Work out the finished part from the listing and answer in its coordinate system (mm). A direction names the side the tool comes from. Coordinates: 2 decimals unless noted, no trailing zeros. Order: outer loops, then holes, each group sorted by start corner. A loop starts at its lowest first (then second) coordinate and runs counter-clockwise, first axis right, second up. Notation, with made-up numbers: M 59.5,-24 L 108.5,-24 A21 cw 108.5,-18 Z; hole C -0.5,-25 d11. An arc over 180 degrees is marked long. Use a Markdown table: item, result. Add a question column.
from build123d import *

# Parameters (mm, degrees)
ESQUISSE1_W              = 86
ESQUISSE1_H              = 40
BOSS_EXTRU_1_DEPTH       = 4
ESQUISSE2_R              = 10.5
ENL_V_MAT_EXTRU_1_DEPTH  = 95.93155429
ESQUISSE3_W              = 6
ESQUISSE3_H              = 40
BOSS_EXTRU_2_DEPTH       = 120
ESQUISSE4_W              = 40
ESQUISSE4_H              = 5
BOSS_EXTRU_3_DEPTH       = 20
ESQUISSE5_W              = 40
ESQUISSE5_H              = 5
BOSS_EXTRU_4_DEPTH       = 20
D_GAGEMENT_M51_D         = 5.5
ESQUISSE32_W             = 40
ESQUISSE32_H             = 31
BOSS_EXTRU_5_DEPTH       = 29.5
ESQUISSE33_W             = 40
ESQUISSE33_H             = 31
BOSS_EXTRU_6_DEPTH       = 29.5
ESQUISSE39_R             = 1.5
ENL_V_MAT_EXTRU_4_DEPTH  = 168.964281917
ESQUISSE43_W             = 30
ESQUISSE43_H             = 31
ENL_V_MAT_EXTRU_12_DEPTH = 29.5
ESQUISSE44_W             = 30
ESQUISSE44_H             = 31
ENL_V_MAT_EXTRU_13_DEPTH = 29.5
ENL_V_MAT_EXTRU_14_DEPTH = 166.033329967
ESQUISSE47_R             = 1.75
ESQUISSE47_R_2           = 1.7
ENL_V_MAT_EXTRU_15_DEPTH = 168.964281917


with BuildPart() as part:
    # Esquisse1 → Boss.-Extru.1 (new body)
    with BuildSketch(Plane(origin=(0, 0, 0), x_dir=(1, 0, 0), z_dir=(0, 1, 0))):
        with Locations((43, 20)):
            Rectangle(ESQUISSE1_W, ESQUISSE1_H)
    extrude(amount=BOSS_EXTRU_1_DEPTH)

    # Esquisse2 → Enlèv. mat.-Extru.1 (cut, through all)
    with BuildSketch(Plane(origin=(0, 4, 0), x_dir=(1, 0, 0), z_dir=(0, 1, 0))):
        with Locations(Location((43, 20, 0), (0, 0, 270))):
            Circle(ESQUISSE2_R)
    extrude(amount=-ENL_V_MAT_EXTRU_1_DEPTH, mode=Mode.SUBTRACT)

    # Esquisse3 → Boss.-Extru.2 (add)
    with BuildSketch(Plane(origin=(0, 0, 0), x_dir=(-1, 0, 0), z_dir=(0, -1, 0))):
        with Locations((-3, 20)):
            Rectangle(ESQUISSE3_W, ESQUISSE3_H)
        with Locations((-83, 20)):
            Rectangle(ESQUISSE3_W, ESQUISSE3_H)
    extrude(amount=BOSS_EXTRU_2_DEPTH)

    # Esquisse4 → Boss.-Extru.3 (add)
    with BuildSketch(Plane.ZY):
        with Locations((-20, -117.5)):
            Rectangle(ESQUISSE4_W, ESQUISSE4_H)
    extrude(amount=BOSS_EXTRU_3_DEPTH)

    # Esquisse5 → Boss.-Extru.4 (add)
    with BuildSketch(Plane(origin=(86, 0, 0), x_dir=(0, 0, -1), z_dir=(1, 0, 0))):
        with Locations((20, -117.5)):
            Rectangle(ESQUISSE5_W, ESQUISSE5_H)
    extrude(amount=BOSS_EXTRU_4_DEPTH)

    # Dégagement M51 (through all)
    with Locations(Plane(origin=(0, -115, 0), x_dir=(1, 0, 0), z_dir=(0, 1, 0))):
        with Locations((-10, 32), (-10, 8), (96, 32), (96, 8)):
            Hole(D_GAGEMENT_M51_D / 2)

    # Esquisse32 → Boss.-Extru.5 (add)
    with BuildSketch(Plane(origin=(6, 0, 0), x_dir=(0, 0, -1), z_dir=(1, 0, 0))):
        with Locations((20, -15.5)):
            Rectangle(ESQUISSE32_W, ESQUISSE32_H)
    extrude(amount=BOSS_EXTRU_5_DEPTH)

    # Esquisse33 → Boss.-Extru.6 (add)
    with BuildSketch(Plane.ZY.offset(-80)):
        with Locations((-20, -15.5)):
            Rectangle(ESQUISSE33_W, ESQUISSE33_H)
    extrude(amount=BOSS_EXTRU_6_DEPTH)

    # Esquisse39 → Enlèv. mat.-Extru.4 (cut, through all)
    with BuildSketch(Plane(origin=(0, 4, 0), x_dir=(1, 0, 0), z_dir=(0, 1, 0))):
        with Locations(Location((33.410152006, 28.776947958, 0), (0, 0, 270))):
            Circle(ESQUISSE39_R)
        with Locations(Location((33.410152006, 11.223052042, 0), (0, 0, 270))):
            Circle(ESQUISSE39_R)
        with Locations(Location((52.589847994, 11.223052042, 0), (0, 0, 270))):
            Circle(ESQUISSE39_R)
        with Locations(Location((52.589847994, 28.776947958, 0), (0, 0, 270))):
            Circle(ESQUISSE39_R)
    extrude(amount=-ENL_V_MAT_EXTRU_4_DEPTH, mode=Mode.SUBTRACT)

    # Esquisse43 → Enlèv. mat.-Extru.12 (cut)
    with BuildSketch(Plane(origin=(35.5, 0, 0), x_dir=(0, 0, -1), z_dir=(1, 0, 0))):
        with Locations((20, -15.5)):
            Rectangle(ESQUISSE43_W, ESQUISSE43_H)
    extrude(amount=-ENL_V_MAT_EXTRU_12_DEPTH, mode=Mode.SUBTRACT)

    # Esquisse44 → Enlèv. mat.-Extru.13 (cut)
    with BuildSketch(Plane.ZY.offset(-50.5)):
        with Locations((-20, -15.5)):
            Rectangle(ESQUISSE44_W, ESQUISSE44_H)
    extrude(amount=-ENL_V_MAT_EXTRU_13_DEPTH, mode=Mode.SUBTRACT)

    # Esquisse34 → Enlèv. mat.-Extru.14 (cut, through all)
    with BuildSketch(Plane.XY):
        Polygon((6, -31), (35.5, 0), (35.5, -31), align=None)
        Polygon((50.5, 0), (80, -31), (50.5, -31), align=None)
    extrude(amount=-ENL_V_MAT_EXTRU_14_DEPTH, mode=Mode.SUBTRACT)

    # Esquisse47 → Enlèv. mat.-Extru.15 (cut, through all)
    with BuildSketch(Plane(origin=(0, 4, 0), x_dir=(1, 0, 0), z_dir=(0, 1, 0))):
        with Locations(Location((9.5, 20, 0), (0, 0, 270))):
            Circle(ESQUISSE47_R)
        with Locations(Location((76.5, 20, 0), (0, 0, 270))):
            Circle(ESQUISSE47_R_2)
    extrude(amount=-ENL_V_MAT_EXTRU_15_DEPTH, mode=Mode.SUBTRACT)


solid = part.part
(1) A cutting plane is placed at C-C on z = -20. Write down the section's boundary in (x, y), plus the area to 3 significant figures.
(2) Straight lines are drawn through the part: line 1 (X direction, y = -116.15, z = -32); line 2 (X direction, y = 1, z = -20); line 3 (X direction, y = -23.5, z = -32.5). For each, find the intervals that lie inside material, in ascending order.
(3) Given P1, Ø2.5, axis at x = 52.59, z = -28.78, coming from the +Y side; P2, Ø9, axis at x = 96, z = -8, coming from the +Y side; P3, Ø12, axis at x = 87, z = -5.5, coming from the +Y side; P4, Ø3, axis at y = -62.5, z = -8, coming from the -X side, each flat-ended and moving along its own axis, determine where each tip first touches the part or whether it passes through.
(4) A cutting plane is placed at A-A on x = 96. Write down the section's boundary in (y, z).
(5) The mould has two halves that part along X. Classify faces 1 (the flat face through (6, -59, -20)), 2 (the flat face through (6, -30.7, 0)), 3 (the flat face through (86, -56, -20)): pulls with the +X half, pulls with the -X half, needs draft (parallel to the pull), parting line crosses it, or undercut.
(6) Which of the six approach directions +Z, -Z, +X, -X, +Y, -Y give full straight-line access (tool end or side, diameter ignored) to faces 4 (the flat face through (-10, -115, -20)), 5 (the flat face through (-7, -120, -20)), 6 (the flat face through (14, -9, -5)), 7 (the flat face through (20.54, -15.72, -2.46)), 8 (the cylindrical face through (33.685, 2.028, -15.155))?
(7) A cutting plane is placed at B-B on y = -47.5. Write down the section's boundary in (x, z), plus the area to 3 significant figures.
(8) A cutting plane is placed at D-D on x = 43. Write down the section's boundary in (y, z), plus the area to 3 significant figures.
From the geometry:
| question | item | result |
|---|---|---|
| 1 | outline | M -20,-120 L 6,-120 L 6,0 L 7.75,0 L 7.75,4 L 0,4 L 0,-115 L -20,-115 Z; M 11.25,0 L 32.5,0 L 32.5,4 L 11.25,4 Z; M 53.5,0 L 74.8,0 L 74.8,4 L 53.5,4 Z; M 78.2,0 L 80,0 L 80,-120 L 106,-120 L 106,-115 L 86,-115 L 86,4 L 78.2,4 Z |
| 1 | area | 1,870 mm2 |
| 2 | line 1 | x = -20 to -12.75, -7.25 to 6, 80 to 93.25, 98.75 to 106 |
| 2 | line 2 | x = 0 to 7.75, 11.25 to 32.5, 53.5 to 74.8, 78.2 to 86 |
| 2 | line 3 | x = 0 to 6, 80 to 86 |
| 3 | P1 | passes through |
| 3 | P2 | stops at y = -115 |
| 3 | P3 | stops at y = 4 |
| 3 | P4 | stops at x = 0 |
| 4 | outline | M -120,-40 L -115,-40 L -115,-34.75 L -120,-34.75 Z; M -120,-29.25 L -115,-29.25 L -115,-10.75 L -120,-10.75 Z; M -120,-5.25 L -115,-5.25 L -115,0 L -120,0 Z |
| 5 | face 1 | undercut |
| 5 | face 2 | needs draft |
| 5 | face 3 | pulls with the +X half |
| 6 | face 4 | +Z, -Z, -X, +Y |
| 6 | face 5 | +Z, -Z, +X, -X, -Y |
| 6 | face 6 | -Y |
| 6 | face 7 | +Z, -Z, -Y |
| 6 | face 8 | +Y, -Y |
| 7 | outline | M 0,-40 L 6,-40 L 6,0 L 0,0 Z; M 80,-40 L 86,-40 L 86,0 L 80,0 Z |
| 7 | area | 480 mm2 |
| 8 | outline | M 0,-40 L 4,-40 L 4,-30.5 L 0,-30.5 Z; M 0,-9.5 L 4,-9.5 L 4,0 L 0,0 Z |
| 8 | area | 76.0 mm2 |
